```python
from build123d import *

# Parameters (mm, degrees)
BOSS_EXTRUDE1_DEPTH      = 25.4
SKETCH2_R                = 1.5875
CUT_EXTRUDE1_DEPTH       = 26.4
SKETCH3_W                = 12.7
SKETCH3_H                = 19.05
CUT_EXTRUDE2_DEPTH       = 19.05
F_5_16_24_TAPPED_HOLE1_D = 6.9088


with BuildPart() as part:
    # Sketch1 → Boss-Extrude1 (new body)
    with BuildSketch(Plane(origin=(0, 0, 0), x_dir=(0, 0, -1), z_dir=(1, 0, 0))):
        Polygon((0, 0), (0, 63.5), (-12.7, 63.5), (-12.7, 19.05), (-31.75, 19.05), (-31.75, 0), align=None)
    extrude(amount=BOSS_EXTRUDE1_DEPTH)

    # Sketch2 → Cut-Extrude1 (cut, through all)
    with BuildSketch(Plane(origin=(25.4, 0, 0), x_dir=(0, 0, -1), z_dir=(1, 0, 0))):
        with Locations((-22.225, 9.525)):
            Circle(SKETCH2_R)
    extrude(amount=-CUT_EXTRUDE1_DEPTH, mode=Mode.SUBTRACT)

    # Sketch3 → Cut-Extrude2 (cut)
    with BuildSketch(Plane.XY.offset(31.75)):
        with Locations((12.7, 9.525)):
            Rectangle(SKETCH3_W, SKETCH3_H)
    extrude(amount=-CUT_EXTRUDE2_DEPTH, mode=Mode.SUBTRACT)

    # 5/16-24 Tapped Hole1 (through all)
    with Locations(Plane(origin=(0, 63.5, 0), x_dir=(1, 0, 0), z_dir=(0, 1, 0))):
        with Locations((12.7, -6.35)):
            Hole(F_5_16_24_TAPPED_HOLE1_D / 2)


solid = part.part
```
Verification items for the finished model (mm, model axes). A direction names the side the tool comes from. Coordinates: 2 decimals unless noted, no trailing zeros. Loops run counter-clockwise (first coordinate to the right, second up) from the corner with the lowest first, then second, coordinate; pieces in that order, holes last. Notation, with made-up numbers: (88.25, 51) -> (136.25, 51) arc R17 cw to (136.25, 66) -> close; hole circle Ø2 at (87.5, 69). An arc over 180 degrees is marked (long way). Answer in a Markdown table with one row per item. Add a question column.
1. Section check C-C, the plane x = 12.7. Enter the section's corners in (y, z).
2. Access from +Z, -Z, +X, -X, +Y, -Y to the whole of each face (thin tool, end or side, straight path). Record for faces 4 (the face through (3, 19.05, 22)), 5 (the face through (19.05, 9, 24)), 6 (the face through (25.4, 25, 9)).
3. Section check D-D, the plane x = 7. Enter the section's corners in (y, z), then the cut area to 3 significant figures.
4. Draft check along Z on faces 1 (the face through (9.405, 31.305, 5.312)), 2 (the face through (3, 10, 31.75)), 3 (the face through (6.35, 9, 24)). Enter one of: +Z half, -Z half, draft (parallel to the pull), parting line (faces both ways), or undercut.
5. Material ranges on probe 1 along Z at (x, y) = (12.7, 19); probe 2 along X at (y, z) = (14, 29); probe 3 along Z at (x, y) = (20.5, 35), recorded low to high. Write a range as [from, to].
6. Section check B-B, the plane y = 50. Enter the section's corners in (x, z).
7. Section check A-A, the plane z = 13.5. Enter the section's corners in (x, y).
8. Depth check by flat-ended pin: P1, Ø1.9, axis at x = 20.5, z = 18, coming from the +Y side. Enter the tip coordinate at first touch or a pass-through.
Derived:
| question | item | result |
|---|---|---|
| 1 | outline | (0, 0) -> (63.5, 0) -> (63.5, 2.9) -> (0, 2.9) -> close; (0, 9.8) -> (63.5, 9.8) -> (63.5, 12.7) -> (0, 12.7) -> close |
| 2 | face 4 | +Z, +X, -X, +Y |
| 2 | face 5 | +Z, +Y, -Y |
| 2 | face 6 | +Z, -Z, +X, +Y, -Y |
| 3 | outline | (0, 0) -> (63.5, 0) -> (63.5, 12.7) -> (0, 12.7) -> close |
| 3 | area | 806 mm² |
| 4 | face 1 | undercut |
| 4 | face 2 | +Z half |
| 4 | face 3 | draft |
| 5 | probe 1 | z = [0, 2.9], [9.8, 12.7] |
| 5 | probe 2 | x = [0, 6.35], [19.05, 25.4] |
| 5 | probe 3 | z = [0, 12.7] |
| 6 | outline | (0, 0) -> (25.4, 0) -> (25.4, 12.7) -> (0, 12.7) -> close; hole circle Ø6.91 at (12.7, 6.35) |
| 7 | outline | (0, 0) -> (6.35, 0) -> (6.35, 19.05) -> (0, 19.05) -> close; (19.05, 0) -> (25.4, 0) -> (25.4, 19.05) -> (19.05, 19.05) -> close |
| 8 | P1 | stops at y = 19.05 |
